Autodesk Inventor part; units mm, degrees
ref_plane "YZ Plane" through (0, 0, 0) normal (1, 0, 0) x (0, 1, 0)
ref_plane "XZ Plane" through (0, 0, 0) normal (0, 1, 0) x (-1, 0, 0)
ref_plane "XY Plane" through (0, 0, 0) normal (0, 0, 1) x (1, 0, 0)
sketch "Block1" plane through (0, 0, 0) normal (0, 0, 1) x (1, 0, 0)
  line L0 (-1.8704, 39.5395) -> (-1.8704, -10.4605)
  line L1 (-4.8704, 39.5395) -> (-4.8704, -10.4605)
  arc A0 (25.8721, -18.7556) -> (25.8721, -22.1655) centre (24.8076, -20.4605) ccw
  arc A1 (25.8721, -28.7556) -> (25.8721, -32.1655) centre (24.8076, -30.4605) ccw
  arc A2 (-25.7569, -32.1655) -> (-25.7569, -28.7556) centre (-24.6924, -30.4605) ccw
  arc A3 (-25.7569, -22.1655) -> (-25.7569, -18.7556) centre (-24.6924, -20.4605) ccw
  line L2 (10.765, -35.4505) -> (20.1076, -35.4505)
  line L3 (20.2076, -15.5605) -> (20.2076, -35.3605)
  line L4 (-20.0924, -15.5605) -> (-20.0924, -35.3605)
  point P0 (0.9099, -18.4595)
sketch "Sketch1" plane through (0, 0, 0) normal (0, 0, 1) x (1, 0, 0)
  circle A0 centre (24.8076, -18.2882) radius 1
  circle A1 centre (24.8076, -28.2882) radius 1
  circle A2 centre (-24.6924, -28.2882) radius 1
  circle A3 centre (-24.6924, -18.2882) radius 1
  line L0 (20.7076, -13.3882) -> (-20.5924, -13.3882)
  line L1 (-20.5924, -13.3882) -> (-20.5924, -33.7782)
  line L2 (-20.5924, -33.7782) -> (20.7076, -33.7782)
  line L3 (20.7076, -33.7782) -> (20.7076, -13.3882)
  line L4 (27.8076, -37.7782) -> (-27.6924, -37.7782)
  line L5 (-27.6924, -37.7782) -> (-27.6924, 2.6118)
  line L6 (-27.6924, 2.6118) -> (27.8076, 2.6118)
  line L7 (27.8076, 2.6118) -> (27.8076, -37.7782)
  line L8 (-1.8704, -8.2882) -> (-1.8704, -13.3882)
  line L9 (-4.8704, -8.2882) -> (-4.8704, -13.3882)
  line L10 (-27.6924, 2.6118) -> (-7.8704, 2.6118)
  line L11 (-7.8704, 2.6118) -> (-7.8704, -9.3882)
  line L12 (-7.8704, -9.3882) -> (-27.6924, -9.3882)
  line L13 (-27.6924, -9.3882) -> (-27.6924, 2.6118)
  line L14 (27.8076, 2.6118) -> (1.1296, 2.6118)
  line L15 (1.1296, 2.6118) -> (1.1296, -9.3882)
  line L16 (1.1296, -9.3882) -> (27.8076, -9.3882)
  line L17 (27.8076, -9.3882) -> (27.8076, 2.6118)
  line L18 (-1.8704, 41.7118) -> (-1.8704, -8.2882)
  line L19 (-4.8704, 41.7118) -> (-4.8704, -8.2882)
  arc A4 (25.8721, -16.5832) -> (25.8721, -19.9932) centre (24.8076, -18.2882) ccw
  arc A5 (25.8721, -26.5832) -> (25.8721, -29.9932) centre (24.8076, -28.2882) ccw
  arc A6 (-25.7569, -29.9932) -> (-25.7569, -26.5832) centre (-24.6924, -28.2882) ccw
  arc A7 (-25.7569, -19.9932) -> (-25.7569, -16.5832) centre (-24.6924, -18.2882) ccw
  line L20 (10.765, -33.2782) -> (20.1076, -33.2782)
  line L21 (20.2076, -13.3882) -> (20.2076, -33.1882)
  line L22 (-20.0924, -13.3882) -> (-20.0924, -33.1882)
  point P0 (0, 0)
  point P1 (15.4363, -33.2782)
  point P2 (-4.8704, -8.2882)
  point P3 (-4.8704, 2.6118)
  point P4 (-1.8704, 2.6118)
  point P5 (-1.8704, -8.2882)
  dimension "d0" = 2
  dimension "d1" = 2
  dimension "d2" = 2
  dimension "d3" = 2
  dimension "d4" = 0.5
  dimension "d5" = 0.5
  dimension "d6" = 0.5
  dimension "d7" = 3
  dimension "d8" = 3
  dimension "d9" = 3
  dimension "d10" = 3
  dimension "d11" = 12
  dimension "d12" = 12
  dimension "d13" = 4
  dimension "d14" = 4
extrude "Extrusion1" add sketch "Sketch1" along normal blind 20 contours L0 L8 L18 L6 L15 L16 L7 L4 L5 L12 L11 L19 L9 L1 L2 L3
sketch "Sketch2" plane through (-7.8704, -9.3882, 0) normal (-1, 0, 0) x (0, 0, 1)
  line L0 (0, 12) -> (0, 0)
  line L1 (0, 0) -> (20, 0)
  line L2 (20, 12) -> (20, 0)
  line L3 (0, 12) -> (20, 12)
  line L4 (20, 6) -> (0, 6)
  line L5 (0, -4) -> (0, 12)
  circle A0 centre (15, 6) radius 1.75
  circle A1 centre (5, 6) radius 1.75
  point P0 (0, 9.3882)
  dimension "d17" = 3.5
  dimension "d18" = 3.5
  dimension "d19" = 10
  dimension "d20" = 20
  dimension "d21" = 5
extrude "Extrusion2" cut sketch "Sketch2" against normal blind 20 contours A1 L4 | L4 A1 | A0 L4 | L4 A0
fillet "Fillet1" radius 3 4 edges at (27.8076, -9.3882, 10) (27.8076, -37.7782, 10) (-27.6924, -37.7782, 10) (-27.6924, -9.3882, 10)
equation "\"d6\" = d4"
equation "\"d12\" = d11"
properties part number "Servo mount_3DPrint"
Part model, mm, in its own coordinate system. A direction names the side the tool comes from. Round coordinates to 2 decimals unless told otherwise and drop trailing zeros. Write each loop counter-clockwise with the first axis right and the second up, starting at its lowest first coordinate (ties: lowest second). Pieces come first, ordered by that corner, then holes. Notation, with made-up numbers: M 88,44.25 L 146,44.25 A13 ccw 146,62.25 Z; hole C 27.5,-37 d4. An arc over 180 degrees is marked long. Return JSON: item names as keys, results as strings. Group by question number.
(1) Saw through at D-D on z = 15. Count the separate pieces of the cut face and the enclosed holes in it, then the cut area to 3 significant figures.
(2) Which spindle directions (+Z, -Z, +X, -X, +Y, -Y) get a long thin tool onto all of the face, cutting with end or side? Do faces 4 (the face through (10, -13.388, 10)), 5 (the face through (13, -9.388, 10)), 6 (the face through (-16, -9.388, 10)), 7 (the face through (27.808, -23, 10)), 8 (the face through (-4.87, -5, 10)). Say none if no direction does.
(3) Saw through at A-A on x = -7. Write the cut outline in (y, z), then the cut area to 3 significant figures.
(4) Saw through at B-B on y = -33. Write the cut outline in (x, z).
(5) Drill centre lines: probe 1 along X at (y, z) = (-16.5, 5); probe 2 along Y at (x, z) = (9.5, 5.25); probe 3 along X at (y, z) = (-17.5, 14). Where is each one in solid material? Low to high.
(6) Two-plate mould, pull along Z, no slides. Class faces 1 (the face through (0, -13, 20)), 2 (the face through (-13, -13.388, 10)), 3 (the face through (-0.39, -2.86, 16.67)): +Z half, -Z half, draft (parallel to the pull), parting line (faces both ways), or undercut.
(7) Saw through at C-C on x = 13. Write the cut outline in (y, z).
(8) Pin check, flat tips, straight feed: pin 1 Ø3 at (y, z) = (-3.39, 15) entering from +X; pin 2 Ø10 at (x, y) = (-5, -16.5) entering from +Z; pin 3 Ø6 at (x, z) = (19, 13.5) entering from +Y; pin 4 Ø6 at (y, z) = (-5.5, 9.5) entering from -X. Stop position of each tip, or through.
Returned:
{
 "1": {"separate pieces": "3", "enclosed holes": "4", "area": "752 mm²"},
 "2": {"face 4": "+Z, -Z", "face 5": "+Z, -Z, +X, +Y", "face 6": "+Z, -Z, -X, +Y", "face 7": "+Z, -Z, +X, +Y, -Y", "face 8": "+Z, -Z, +Y"},
 "3": {"outline": "M -37.78,0 L -33.78,0 L -33.78,20 L -37.78,20 Z; M -13.39,0 L 2.61,0 L 2.61,20 L -13.39,20 Z; hole C -3.39,5 d3.5; hole C -3.39,15 d3.5", "area": "381 mm²"},
 "4": {"outline": "M -27.69,0 L -20.59,0 L -20.59,20 L -27.69,20 Z; M 20.71,0 L 27.81,0 L 27.81,20 L 20.71,20 Z"},
 "5": {"probe 1": "-27.69 to -20.59, 20.71 to 27.81", "probe 2": "-37.78 to -33.78, -13.39 to -9.39", "probe 3": "-27.69 to -25.31, -24.08 to -20.59, 20.71 to 24.19, 25.42 to 27.81"},
 "6": {"face 1": "+Z half", "face 2": "draft", "face 3": "undercut"},
 "7": {"outline": "M -37.78,0 L -33.78,0 L -33.78,20 L -37.78,20 Z; M -13.39,0 L -9.39,0 L -9.39,20 L -13.39,20 Z"},
 "8": {"pin 1": "through", "pin 2": "z = 20", "pin 3": "y = -9.39", "pin 4": "x = -7.87"}
}
